Could you check a few things on this model? Use its own coordinates, in mm. A direction names the side the tool comes from. Round coordinates to 2 decimals unless told otherwise and drop trailing zeros. Write each loop counter-clockwise with the first axis right and the second up, starting at its lowest first coordinate (ties: lowest second). Pieces come first, ordered by that corner, then holes. Notation, with made-up numbers: (37, -37.75) -> (82, -37.75) arc R29 ccw to (82, -15.75) -> close; hole circle Ø11 at (-16, 85.5). An arc over 180 degrees is marked (long way). One line per question, with ' | ' between items. Start each with the question number.
1. Imagine slicing it at D-D, the plane y = -15.5. List the corners of the cut face in (x, z) for me, and give its area (3 significant figures).
2. Imagine slicing it at B-B, the plane x = 15.5. List the corners of the cut face in (y, z) for me (3 decimals), and give its area (3 significant figures).
3. Imagine slicing it at A-A, the plane y = 0. List the corners of the cut face in (x, z) for me, and give its area (3 significant figures).
4. For pin 1 Ø8 at (x, y) = (-14.5, -7) entering from +Z; pin 2 Ø2.5 at (x, z) = (1, 6) entering from -Y; pin 3 Ø3.5 at (x, y) = (-0.5, -23) entering from +Z; pin 4 Ø6 at (x, y) = (0, 0) entering from +Z, each with a flat end and sliding along its axis, tell me the tip position at first contact or that it passes through.
5. If I drill on line 1 along X through (y, z) = (-15.5, 1.35); line 2 along Y through (x, z) = (0, 1.35) (3 decimals); line 3 along Y through (x, z) = (-3.5, 4.25) (3 decimals), over which ranges is the centre line in solid material (lowest first)? Write a range as [from, to].
6. Imagine slicing it at C-C, the plane z = 0.75. List the corners of the cut face in (x, y) for me (3 decimals), and give its area (3 significant figures).
7. For faces 4 (the flat face through (0, 6, 0)), 5 (the flat face through (-0.3, -22, 3.8)), 6 (the flat face through (0, -24, 4)), which set-ups out of +Z, -Z, +X, -X, +Y, -Y let a thin tool reach every point of the face, with its end or its side?
8. Thinking about a two-plate mould opening in X: for faces 1 (the cylindrical face through (15.43, -14, 1.48)), 2 (the flat face through (-24, 0, 4)), 3 (the flat face through (0, 25.175, 4)), which applies, released by +X, released by -X, zero draft, split by the parting line, or undercut?
Autodesk Inventor part; units mm, degrees
ref_plane "YZ Plane" through (0, 0, 0) normal (1, 0, 0) x (0, 1, 0)
ref_plane "XZ Plane" through (0, 0, 0) normal (0, 1, 0) x (-1, 0, 0)
ref_plane "XY Plane" through (0, 0, 0) normal (0, 0, 1) x (1, 0, 0)
sketch "Sketch1" plane through (0, 0, 0) normal (0, 0, 1) x (1, 0, 0)
  line L0 (0, 0) -> (22, 0)
  line L1 (22, 0) -> (22, 22)
  line L2 (22, 22) -> (-22, 22)
  line L3 (-22, 22) -> (-22, -22)
  line L4 (-22, -22) -> (22, -22)
  line L5 (22, -22) -> (22, 22)
  line L6 (-22, 22) -> (-22, 25.175)
  line L7 (-22, 25.175) -> (-25.175, 25.175)
  line L8 (22, -22) -> (25.175, -22)
  line L9 (25.175, -22) -> (25.175, -25.175)
  line L10 (-25.175, 25.175) -> (25.175, 25.175)
  line L11 (25.175, 25.175) -> (25.175, -25.175)
  line L12 (25.175, -25.175) -> (-25.175, -25.175)
  line L13 (-25.175, -25.175) -> (-25.175, 25.175)
  dimension "d0" = 22
  dimension "d1" = 22
  dimension "d2" = 44
  dimension "d3" = 44
  dimension "d4" = 3.175
  dimension "d5" = 3.175
  dimension "d6" = 3.175
  dimension "d7" = 3.175
extrude "Extrusion1" add sketch "Sketch1" along normal blind 8 contours L1 L2 L6 L10 L11 L8 L5 | L8 L9 L12 L13 L7 L6 L3 L4
sketch "Sketch2" plane through (0, 0, 0) normal (0, 0, -1) x (-1, 0, 0)
  line L0 (22, 22) -> (-22, 22)
  line L1 (-22, 22) -> (-22, -22)
  line L2 (22, 22) -> (-22, 22)
  line L3 (-22, 22) -> (-22, -22)
  line L4 (-22, -22) -> (22, -22)
  line L5 (22, -22) -> (22, 22)
  point P0 (0, 0)
extrude "Extrusion2" add sketch "Sketch2" against normal blind 3
sketch "Sketch3" plane through (0, 0, 3) normal (0, 0, 1) x (1, 0, 0)
  line L0 (-22, 22) -> (22, 22)
  line L1 (-22, 22) -> (0, 22)
  point P0 (0, 0)
  point P1 (0, 0)
hole "Hole1" at (0, 0, 3) direction (0, 0, -1) diameter 10 end through all
sketch "Sketch4" plane through (0, 0, 3) normal (0, 0, 1) x (1, 0, 0)
  line L0 (0, 0) -> (0, 15.5)
  line L1 (0, 15.5) -> (15.5, 15.5)
  line L2 (15.5, 15.5) -> (-15.5, 15.5)
  line L3 (-15.5, 15.5) -> (-15.5, -15.5)
  line L4 (-15.5, -15.5) -> (15.5, -15.5)
  line L5 (15.5, -15.5) -> (15.5, 15.5)
  dimension "d19" = 15.5
  dimension "d20" = 15.5
  dimension "d21" = 31
  dimension "d22" = 31
hole "Hole2" at (-15.5, 15.5, 3) at (15.5, 15.5, 3) at (15.5, -15.5, 3) at (-15.5, -15.5, 3) direction (0, 0, -1) diameter 3 end through all
sketch "Sketch5" plane through (0, 0, 8) normal (0, 0, 1) x (1, 0, 0)
  line L0 (22, 22) -> (22, -22)
  line L1 (22, -22) -> (22, -25.175)
  line L2 (-25.175, -25.175) -> (25.175, -25.175)
  line L3 (22, -25.175) -> (24, -25.175)
  line L4 (22, -22) -> (-22, -22)
  line L5 (-22, -22) -> (-22, -25.175)
  line L6 (-22, -25.175) -> (-24, -25.175)
  line L7 (25.175, -25.175) -> (25.175, 25.175)
  line L8 (24, -25.175) -> (25.175, -25.175)
  line L9 (25.175, -25.175) -> (25.175, 25.175)
  line L10 (25.175, 25.175) -> (24, 25.175)
  line L11 (24, 25.175) -> (24, -25.175)
  line L12 (25.175, 25.175) -> (-25.175, 25.175)
  line L13 (-24, -25.175) -> (-25.175, -25.175)
  line L14 (-25.175, -25.175) -> (-25.175, 25.175)
  line L15 (-25.175, 25.175) -> (-24, 25.175)
  line L16 (-24, 25.175) -> (-24, -25.175)
  point P0 (0, 0)
  dimension "d30" = 2
  dimension "d31" = 2
extrude "Extrusion3" cut sketch "Sketch5" against normal blind 8 contours L11 L10 L7 L2 | L2 L14 L12 L16
sketch "Sketch6" plane through (0, 0, 8) normal (0, 0, 1) x (1, 0, 0)
  line L0 (22, -22) -> (-22, -22)
  line L1 (-24, -25.175) -> (24, -25.175)
  line L2 (0, -22) -> (-4, -22)
  line L3 (-4, -22) -> (-4, -25.175)
  line L4 (-4, -25.175) -> (0, -25.175)
  line L5 (0, -25.175) -> (0, -22)
  line L6 (0, -22) -> (4, -22)
  line L7 (4, -22) -> (4, -25.175)
  line L8 (4, -25.175) -> (0, -25.175)
  line L9 (0, -25.175) -> (0, -22)
  point P0 (0, 0)
  dimension "d34" = 4
  dimension "d35" = 4
extrude "Extrusion4" cut sketch "Sketch6" against normal blind 4
fillet "Fillet1" radius 2 2 edges at (-4, -23.5875, 4) (4, -23.5875, 4)
properties part number "RollMotorMount"
Geometry results:
1) outline: (-24, 0) -> (-17, 0) -> (-17, 3) -> (-22, 3) -> (-22, 8) -> (-24, 8) -> close; (-14, 0) -> (14, 0) -> (14, 3) -> (-14, 3) -> close; (17, 0) -> (24, 0) -> (24, 8) -> (22, 8) -> (22, 3) -> (17, 3) -> close | area: 146 mm2
2) outline: (-25.175, 0) -> (-17, 0) -> (-17, 3) -> (-22, 3) -> (-22, 8) -> (-25.175, 8) -> close; (-14, 0) -> (14, 0) -> (14, 3) -> (-14, 3) -> close; (17, 0) -> (25.175, 0) -> (25.175, 8) -> (22, 8) -> (22, 3) -> (17, 3) -> close | area: 165 mm2
3) outline: (-24, 0) -> (-5, 0) -> (-5, 3) -> (-22, 3) -> (-22, 8) -> (-24, 8) -> close; (5, 0) -> (24, 0) -> (24, 8) -> (22, 8) -> (22, 3) -> (5, 3) -> close | area: 134 mm2
4) pin 1: stops at z = 3 | pin 2: stops at y = 22 | pin 3: stops at z = 4.02 | pin 4: passes through
5) line 1: x = [-24, -17], [-14, 14], [17, 24] | line 2: y = [-25.175, -5], [5, 25.175] | line 3: y = [-25.175, -22], [22, 25.175]
6) outline: (-24, -25.175) -> (24, -25.175) -> (24, 25.175) -> (-24, 25.175) -> close; hole circle Ø3 at (-15.5, -15.5); hole circle Ø3 at (-15.5, 15.5); hole circle Ø10 at (0, 0); hole circle Ø3 at (15.5, -15.5); hole circle Ø3 at (15.5, 15.5) | area: 2,310 mm2
7) face 4: -Z, +X, -X, +Y, -Y | face 5: +Z | face 6: +Z, -Y
8) face 1: undercut | face 2: released by -X | face 3: zero draft
